```python
from build123d import *

# Parameters (mm, degrees)
F0_W     = 100
F0_H     = 80
F1_DEPTH = 10
F3_D     = 10
F4_R     = 5
F5_R     = 5
F6_W     = 80
F6_H     = 10
F7_DEPTH = 80
F8_SIZE  = 10
F10_D    = 40


with BuildPart() as f1:
    # F0 (on Top) → F1 (new body)
    with BuildSketch(Plane.XY):
        with Locations((13.55473, -5.91478)):
            Rectangle(F0_W, F0_H)
    extrude(amount=F1_DEPTH)

    # F3 (through all)
    with Locations(Plane.XY.offset(10)):
        with Locations((-21.44527, -30.91478), (-21.44527, 19.08522), (48.55473, 19.08522), (48.55473, -30.91478)):
            Hole(F3_D / 2)

    # F4
    f4_edges = [f1.edges().sort_by_distance(p)[0] for p in [
        (63.55473, 34.08522, 5),
    ]]
    fillet(f4_edges, radius=F4_R)

    # F5
    f5_edges = [f1.edges().sort_by_distance(p)[0] for p in [
        (63.55473, -45.91478, 5),
        (-36.44527, -45.91478, 5),
        (-36.44527, 34.08522, 5),
    ]]
    fillet(f5_edges, radius=F5_R)

    # F6 (on face) → F7 (join)
    with BuildSketch(Plane.XY.offset(10)):
        with Locations((13.55473, -5)):
            Rectangle(F6_W, F6_H)
    extrude(amount=F7_DEPTH)

    # F8
    f8_edges = [f1.edges().sort_by_distance(p)[0] for p in [
        (53.55473, -5, 90),
        (-26.44527, -5, 90),
    ]]
    chamfer(f8_edges, length=F8_SIZE)

    # F10 (through all)
    with Locations(Plane.XZ.offset(10)):
        with Locations((12.048366, 50.624441)):
            Hole(F10_D / 2)


solid = f1.part
```
Geometry check sheet. Reference: the model listing, model coordinates, mm. A direction names the side the tool comes from. Round coordinates to 2 decimals unless told otherwise and drop trailing zeros. Order: outer loops, then holes, each group sorted by start corner. A loop starts at its lowest first (then second) coordinate and runs counter-clockwise, first axis right, second up. Notation, with made-up numbers: (81.25, 84) - (97.25, 84) arc R24 ccw to (97.25, 121) - close; hole circle Ø3 at (25.5, 22.25). An arc over 180 degrees is marked (long way). Use a Markdown table: item, result. Add a question column.
(1) Sectioned sample at A-A, the plane z = 8. Enter the section's corners in (x, y).
(2) Depth check by flat-ended pin: pin 1 (2 mm diameter, centred on x = 50, z = 61.5, fed in from -Y); pin 2 (8 mm diameter, centred on x = 46, y = -28, fed in from +Z); pin 3 (11 mm diameter, centred on y = -7, z = 47.5, fed in from -X). Enter the tip coordinate at first touch or a pass-through.
(3) Sectioned sample at D-D, the plane y = 21.5. Enter the section's corners in (x, z).
(4) Tool access check on faces 5 (the flat face through (53.555, -5, 45)), 6 (the cylindrical face through (-34.9, 32.7, 5.1)). Record the directions out of +Z, -Z, +X, -X, +Y, -Y that give a thin tool (end or side, any length) a straight path to the whole face; none if there is none.
(5) Sectioned sample at B-B, the plane x = 13. Enter the section's corners in (y, z), and give its area (3 significant figures).
(6) Sectioned sample at C-C, the plane x = -12.5. Enter the section's corners in (y, z).
(7) Material ranges on line 1 along Z through (x, y) = (13, -3.5); line 2 along X through (y, z) = (21.5, 6); line 3 along Y through (x, z) = (2, 26), recorded low to high. Write a range as [from, to].
(8) Release check for a two-part mould opening along Y. For faces 1 (the flat face through (22, 0, 32)), 2 (the cylindrical face through (43.786, 20.587, 4.93)), 3 (the flat face through (-26.445, -5, 45)), 4 (the cylindrical face through (-20.361, -35.796, 4.93)) record: pulls with the +Y half, pulls with the -Y half, needs draft (parallel to the pull), parting line crosses it, or undercut.
Answers below:
| question | item | result |
|---|---|---|
| 1 | outline | (-36.45, -40.91) arc R5 ccw to (-31.45, -45.91) - (58.55, -45.91) arc R5 ccw to (63.55, -40.91) - (63.55, 29.09) arc R5 ccw to (58.55, 34.09) - (-31.45, 34.09) arc R5 ccw to (-36.45, 29.09) - close; hole circle Ø10 at (-21.45, -30.91); hole circle Ø10 at (-21.45, 19.09); hole circle Ø10 at (48.55, -30.91); hole circle Ø10 at (48.55, 19.09) |
| 2 | pin 1 | y = -10 |
| 2 | pin 2 | z = 10 |
| 2 | pin 3 | x = -26.45 |
| 3 | outline | (-36.45, 0) - (-25.82, 0) - (-25.82, 10) - (-36.45, 10) - close; (-17.07, 0) - (44.18, 0) - (44.18, 10) - (-17.07, 10) - close; (52.93, 0) - (63.55, 0) - (63.55, 10) - (52.93, 10) - close |
| 4 | face 5 | +Z, +X, +Y, -Y |
| 4 | face 6 | +Z, -Z, -X, +Y |
| 5 | outline | (-45.91, 0) - (34.09, 0) - (34.09, 10) - (0, 10) - (0, 30.65) - (-10, 30.65) - (-10, 10) - (-45.91, 10) - close; (-10, 70.6) - (0, 70.6) - (0, 90) - (-10, 90) - close |
| 5 | area | 1,200 mm² |
| 6 | outline | (-45.91, 0) - (34.09, 0) - (34.09, 10) - (0, 10) - (0, 90) - (-10, 90) - (-10, 10) - (-45.91, 10) - close |
| 7 | line 1 | [0, 30.65], [70.6, 90] |
| 7 | line 2 | [-36.45, -25.82], [-17.07, 44.18], [52.93, 63.55] |
| 7 | line 3 | [-10, 0] |
| 8 | face 1 | pulls with the +Y half |
| 8 | face 2 | undercut |
| 8 | face 3 | needs draft |
| 8 | face 4 | undercut |
